Build history of the part. All positions in model axes, mm. Round coordinates to 2 decimals unless told otherwise and drop trailing zeros. Write each loop counter-clockwise with the first axis right and the second up, starting at its lowest first coordinate (ties: lowest second). Pieces come first, ordered by that corner, then holes.
Autodesk Inventor part; units mm, degrees
ref_plane "YZ Plane" through (0, 0, 0) normal (1, 0, 0) x (0, 1, 0)
ref_plane "XZ Plane" through (0, 0, 0) normal (0, 1, 0) x (-1, 0, 0)
ref_plane "XY Plane" through (0, 0, 0) normal (0, 0, 1) x (1, 0, 0)
ref_plane "Work Plane1" through (0, 0, 0) normal (0, 0, 1) x (1, 0, 0)
sketch "Sketch1" plane through (0, 0, 0) normal (0, 0, 1) x (1, 0, 0)
  arc A0 (-18.155, 30) -> (-18.155, 0) centre (0, 15) ccw construction
  line L0 (-18.155, 0) -> (-3.4871, 0) construction
  line L1 (-18.155, 30) -> (-3.4871, 30) construction
  circle A1 centre (0, 15) radius 15.4 construction
  arc A2 (-6.5238, 29.25) -> (-6.5238, 0.75) centre (0, 15) ccw construction
  line L2 (-6.5238, 0.75) -> (-17.7982, 0.75) construction
  arc A3 (-17.7982, 29.25) -> (-17.7982, 0.75) centre (0, 15) ccw construction
  line L3 (-17.7982, 29.25) -> (-6.5238, 29.25) construction
  circle A4 centre (0, 15) radius 12.775 construction
  line L4 (-6.5238, 29.25) -> (0, 29.25) construction
  line L5 (-6.5238, 0.75) -> (0, 0.75) construction
  arc A5 (0, 0.75) -> (0, 29.25) centre (0, 15) ccw construction
  line L6 (-42.0841, 29.25) -> (-42.0841, 0.75)
  line L7 (-42.0841, 0.75) -> (0, 0.75)
  line L8 (-42.0841, 29.25) -> (0, 29.25)
  circle A6 centre (0, 15) radius 11.5
  arc A7 (0, 0.75) -> (0, 29.25) centre (0, 15) ccw
  arc A8 (-3.4871, 0) -> (3.4871, 0) centre (0, 15) ccw
  line L9 (3.4871, 0) -> (18, 0)
  line L10 (18, 0) -> (18, 30)
  line L11 (3.4871, 30) -> (18, 30)
  arc A9 (3.4871, 30) -> (-3.4871, 30) centre (0, 15) ccw
  line L12 (-7.3927, 28.5095) -> (7.3927, 28.5095)
  arc A10 (7.3927, 1.4905) -> (7.3927, 28.5095) centre (0, 15) ccw
  line L13 (7.3927, 1.4905) -> (-7.3927, 1.4905)
  arc A11 (-7.3927, 28.5095) -> (-7.3927, 1.4905) centre (0, 15) ccw
  point P0 (0, 0)
  dimension "d0" = 0.75
  dimension "d1" = 25.55
  dimension "d2" = 23
extrude "Extrusion1" add sketch "Sketch1" along normal blind 1 contours L8 A7 L12 A11 L13 L7 L6 | A7 L13 A11 L12
sketch "Sketch2" plane through (0, 0, 1) normal (0, 0, 1) x (1, 0, 0)
  circle A0 centre (0, 15) radius 11.5
  line L0 (0, 29.25) -> (-42.0841, 29.25)
  line L1 (-42.0841, 29.25) -> (-42.0841, 0.75)
  line L2 (-42.0841, 0.75) -> (0, 0.75)
  arc A1 (0, 0.75) -> (0, 29.25) centre (0, 15) ccw
  circle A2 centre (0, 15) radius 12.775
  point P0 (0, 0)
  dimension "d5" = 25.55
extrude "Extrusion2" add sketch "Sketch2" along normal blind 6.25 contours A1 L2 L1 L0
fillet "Rundung1" radius 2 2 edges at (-42.0841, 0.75, 3.625) (-42.0841, 29.25, 3.625)
chamfer "Fasen1" distance 0.4 angle 45 6 edges at (-20.0421, 29.25, 7.25) (-41.4983, 28.6642, 7.25) (-42.0841, 15, 7.25) (-41.4983, 1.3358, 7.25) (-20.0421, 0.75, 7.25) (14.25, 15, 7.25)
chamfer "Fasen2" distance 0.4 angle 45 6 edges at (-20.0421, 0.75, 0) (14.25, 15, 0) (-20.0421, 29.25, 0) (-41.4983, 28.6642, 0) (-42.0841, 15, 0) (-41.4983, 1.3358, 0)
fillet "Rundung2" radius 0.4 1 edges at (-11.5, 15, 0)
fillet "Rundung3" radius 0.4 1 edges at (-11.5, 15, 1)
fillet "Rundung4" radius 0.4 1 edges at (-12.775, 15, 7.25)
properties part number "10_Filteslide_25mm"
1) Slice it at B-B (y = 15). Write the cut outline in (x, z) (3 decimals).
Results:
outline: (-42.084, 0.4) - (-41.684, 0) - (-11.9, 0) arc R0.4 ccw to (-11.5, 0.4) - (-11.5, 0.6) arc R0.4 ccw to (-11.9, 1) - (-12.775, 1) - (-12.775, 6.85) arc R0.4 ccw to (-13.175, 7.25) - (-41.684, 7.25) - (-42.084, 6.85) - close; (11.5, 0.4) arc R0.4 ccw to (11.9, 0) - (13.85, 0) - (14.25, 0.4) - (14.25, 6.85) - (13.85, 7.25) - (13.175, 7.25) arc R0.4 ccw to (12.775, 6.85) - (12.775, 1) - (11.9, 1) arc R0.4 ccw to (11.5, 0.6) - close
2) Mould opens along X. For faces 1 (the flat face through (-27, 15, 7.25)), 2 (the flat face through (-42.084, 15, 4)), 3 (the cylindrical face through (14.247, 15.313, 3.58)), 4 (the cylindrical face through (-1.663, 2.334, 3.884)) say: released by +X, released by -X, zero draft, split by the parting line, or undercut.
Results:
face 1: zero draft
face 2: released by -X
face 3: released by +X
face 4: undercut
3) Wall check: L1, parallel to Y at x = 0, z = 0.5; L2, parallel to Y at x = 0, z = 5.75 (3 decimals); L3, parallel to X at y = 10.5, z = 4.75. Give the ranges that are in metal, low to high.
Results:
L1: y = 0.75 to 3.5, 26.5 to 29.25
L2: y = 0.75 to 2.225, 27.775 to 29.25
L3: x = -42.08 to -11.96, 11.96 to 13.52
4) Pin check, flat tip, straight feed: pin 1 Ø3 at (x, y) = (3, 26) entering from +Z. Stop position of the tip, or through.
Results:
pin 1: stops at z = 7.14
5) Slice it at A-A (z = 2.75). Write the cut outline in (x, y) (3 decimals).
Results:
outline: (-42.084, 2.75) arc R2 ccw to (-40.084, 0.75) - (0, 0.75) arc R14.25 ccw to (0, 29.25) - (-40.084, 29.25) arc R2 ccw to (-42.084, 27.25) - close; hole circle Ø25.55 at (0, 15)
